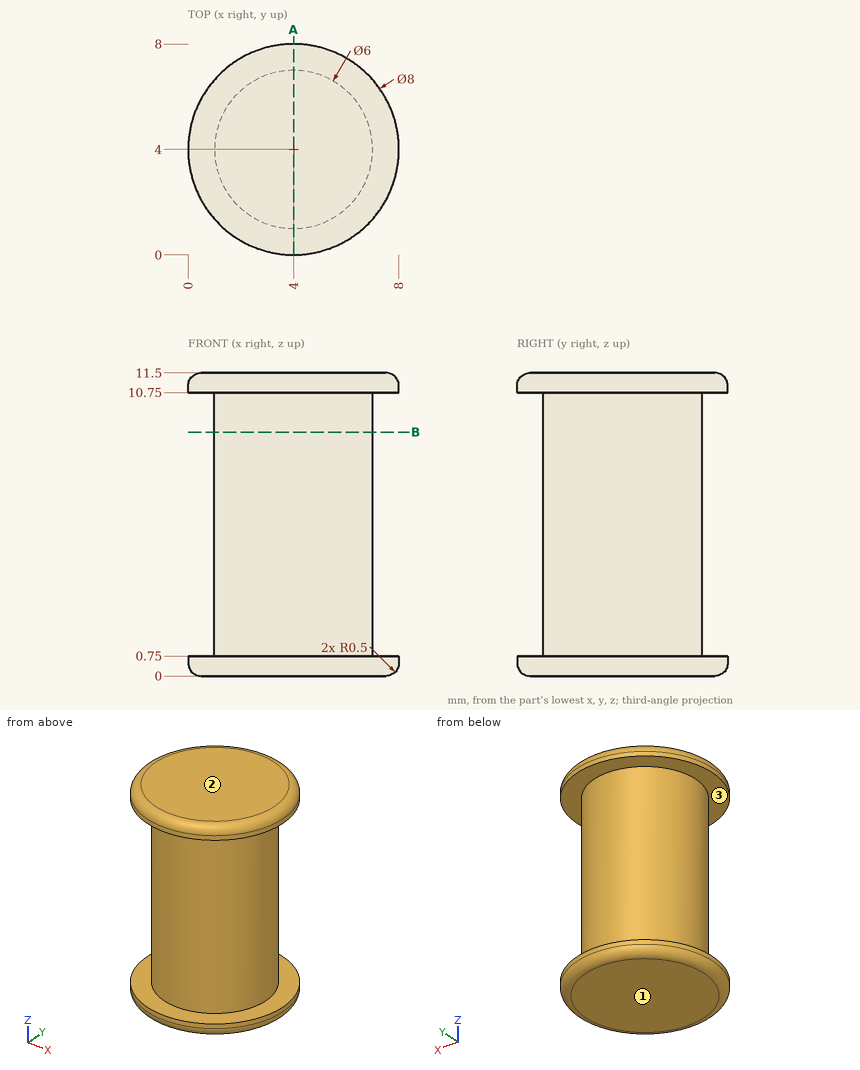
Part print with two shaded views. Sizes in mm from the minimum x, y, z corner. Round coordinates to 2 decimals unless told otherwise and drop trailing zeros. Write each loop counter-clockwise with the first axis right and the second up, starting at its lowest first coordinate (ties: lowest second). Pieces come first, ordered by that corner, then holes. Notation, with made-up numbers: (59.25, 49) -> (95.25, 49) arc R18 ccw to (95.25, 57) -> close; hole circle Ø8 at (58, 21.5). An arc over 180 degrees is marked (long way). Use one line per item in the form item = value.
Q1. Drill centre lines: L1, parallel to Z at x = 1, y = 3.5; L2, parallel to Y at x = 3, z = 1.25; L3, parallel to X at y = 3.75, z = 1.25. Where is each one in solid material? Low to high.
Conclusion:
L1 = 0 to 0.75, 10.75 to 11.5
L2 = 1.17 to 6.83
L3 = 1.01 to 6.99
Q2. Drop flat-ended pins along their axis: P1, Ø1, axis at y = 2, z = 9.5, coming from the +X side; P2, Ø3, axis at y = 4.5, z = 3.5, coming from the -X side; P3, Ø2, axis at x = 2.5, z = 4, coming from the +Y side. Give the stop position or say it passes through.
Conclusion:
P1 = 6.6
P2 = 1
P3 = 6.96
Q3. Band-saw the part on B-B, the plane z = 9.25. Write the cut outline in (x, y).
Conclusion:
outline = circle Ø6 at (4, 4)
Q4. Two-plate mould, pull along Z, no slides. Class the marked faces 1, 2 and 3: released by +Z, released by -Z, zero draft, split by the parting line, or undercut.
Conclusion:
face_1 = released by -Z
face_2 = released by +Z
face_3 = undercut
Q5. Band-saw the part on A-A, the plane x = 4. Write the cut outline in (y, z), then the cut area to 3 significant figures.
Conclusion:
outline = (0, 0.5) arc R0.5 ccw to (0.5, 0) -> (7.5, 0) arc R0.5 ccw to (8, 0.5) -> (8, 0.75) -> (7, 0.75) -> (7, 10.75) -> (8, 10.75) -> (8, 11) arc R0.5 ccw to (7.5, 11.5) -> (0.5, 11.5) arc R0.5 ccw to (0, 11) -> (0, 10.75) -> (1, 10.75) -> (1, 0.75) -> (0, 0.75) -> close
area = 71.8 mm²
